The model under review builds one solid part; all positions refer to its coordinate system, in mm. Face numbers are marked on the shaded views. A direction names the side the tool comes from. Round coordinates to 2 decimals unless told otherwise and drop trailing zeros. Loops run counter-clockwise (first coordinate to the right, second up) from the corner with the lowest first, then second, coordinate; pieces in that order, holes last. Notation, with made-up numbers: (38.25, -21) -> (53.25, -21) arc R16 ccw to (53.25, 2) -> close; hole circle Ø8 at (24.25, 52.5). An arc over 180 degrees is marked (long way). Use a Markdown table: item, result. Add a question column.
1) Wall thickness on probe 1 along X at (y, z) = (24, 0.1); probe 2 along Y at (x, z) = (2.5, -0.05); probe 3 along Y at (x, z) = (1.75, -0.65): over which ranges is each line inside the solid? List them lowest first.
2) Consider section C-C on y = 5. Give the boundary of the cut face in (x, z).
3) Consider section B-B on x = 5.25. Give the boundary of the cut face in (y, z).
4) Consider section A-A on z = 0.4. Give the boundary of the cut face in (x, y).
5) For the marked faces 1, 2 and 3, list the 3-axis set-ups (+Z, -Z, +X, -X, +Y, -Y) from which the entire face can be reached by the end or side of a thin tool; tool diameter is ignored.
from build123d import *

# Parameters (mm, degrees)
SKETCH_1_R      = 0.75
EXTRUDE_1_DEPTH = 38
SKETCH_3_R      = 0.75
EXTRUDE_2_DEPTH = 7
SKETCH_5_R      = 0.75
EXTRUDE_3_DEPTH = 7


with BuildPart() as part:
    # 草图1 → 凸台-拉伸1 (new body)
    with BuildSketch(Plane(origin=(0, 0, 0), x_dir=(1, 0, 0), z_dir=(0, 1, 0))):
        with Locations(Location((0, 0, 0), (0, 0, 270))):
            Circle(SKETCH_1_R)
    extrude(amount=EXTRUDE_1_DEPTH)

    # 草图2 → 旋转1 (revolve)
    with BuildSketch(Plane.XY):
        with BuildLine():
            Line((0, 38.75), (0, 37.25))
            ThreePointArc((0, 37.25), (0.75, 38), (0, 38.75))
        make_face()
    revolve(axis=Axis((0, 38.75, 0), (0, -1, 0)))

    # 草图3 → 凸台-拉伸2 (add)
    with BuildSketch(Plane(origin=(0, 0, 0), x_dir=(0, 0, -1), z_dir=(1, 0, 0))):
        with Locations((0, 38)):
            Circle(SKETCH_3_R)
    extrude(amount=EXTRUDE_2_DEPTH)

    # 草图4 → 旋转2 (revolve)
    with BuildSketch(Plane(origin=(7, 0, 0), x_dir=(0, 0, -1), z_dir=(1, 0, 0))):
        with BuildLine():
            Line((0, 38.75), (0, 37.25))
            ThreePointArc((0, 37.25), (0.75, 38), (0, 38.75))
        make_face()
    revolve(axis=Axis((7, 38.75, 0), (0, -1, 0)))

    # 草图5 → 凸台-拉伸3 (add)
    with BuildSketch(Plane(origin=(0, 38, 0), x_dir=(1, 0, 0), z_dir=(0, 1, 0))):
        with Locations(Location((7, 0, 0), (0, 0, 270))):
            Circle(SKETCH_5_R)
    extrude(amount=EXTRUDE_3_DEPTH)


solid = part.part
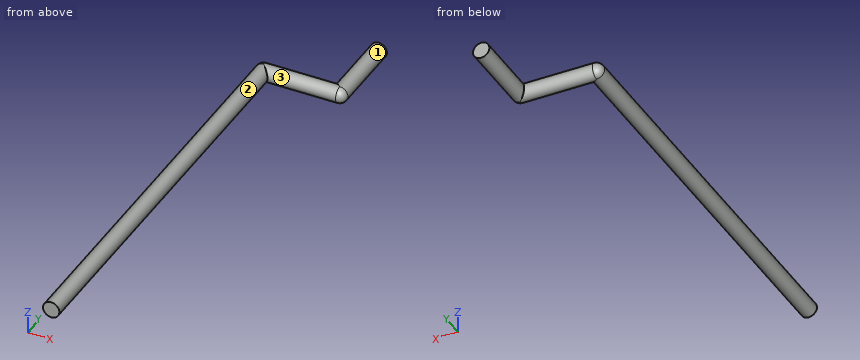
Result set:
| question | item | result |
|---|---|---|
| 1 | probe 1 | -0.74 to 0.74 |
| 1 | probe 2 | 37.25 to 38.75 |
| 1 | probe 3 | 37.63 to 38.37 |
| 2 | outline | circle Ø1.5 at (0, 0) |
| 3 | outline | circle Ø1.5 at (38, 0) |
| 4 | outline | (-0.63, 0) -> (0.63, 0) -> (0.63, 37.37) -> (7, 37.37) arc R0.63 ccw to (7.63, 38) -> (7.63, 45) -> (6.37, 45) -> (6.37, 38.63) -> (0, 38.63) arc R0.63 ccw to (-0.63, 38) -> close |
| 5 | face 1 | +Y |
| 5 | face 2 | -Y |
| 5 | face 3 | none |
